Print and shaded views of the part. All mm, measured from the part's lowest x, y and z. A direction names the side the tool comes from. Coordinates: 2 decimals unless noted, no trailing zeros. Loops run counter-clockwise (first coordinate to the right, second up) from the corner with the lowest first, then second, coordinate; pieces in that order, holes last. Notation, with made-up numbers: M -2.5,-37 L 29.5,-37 A24 cw 29.5,-4 Z; hole C 15,4.25 d5. An arc over 180 degrees is marked long. Use a Markdown table: item, result. Add a question column.
1) Wall check: probe 1 along Y at (x, z) = (51, 8.5); probe 2 along Y at (x, z) = (49.25, 8.5); probe 3 along Z at (x, y) = (3.5, 7.25). Give the ranges that are in metal, low to high. Write a range as from..to.
2) Pull direction Z, two halves, no side cores. Call the marked faces 4, 5 and 6: released by +Z, released by -Z, zero draft, split by the parting line, or undercut.
3) Band-saw the part on B-B (y = 47.69). List the corners of the cut face in (x, z).
4) Band-saw the part on D-D (z = 16.25). List the corners of the cut face in (x, y), plus the area to 3 significant figures.
5) Pin check, flat tips, straight feed: pin 1 Ø5 at (y, z) = (42, 3) entering from -X; pin 2 Ø9 at (x, z) = (13, 10) entering from +Y; pin 3 Ø2 at (x, y) = (7, 7.5) entering from +Z; pin 4 Ø4 at (y, z) = (31, 8.5) entering from -X. Stop position of each tip, or through.
6) Tool access for the marked faces 1, 2 and 3: list every direction of +Z, -Z, +X, -X, +Y, -Y with a clear straight run to the whole face (end or side of a thin tool).
7) Band-saw the part on A-A (z = 8.5). List the corners of the cut face in (x, y), plus the area to 3 significant figures.
8) Band-saw the part on C-C (x = 3.5). List the corners of the cut face in (y, z).
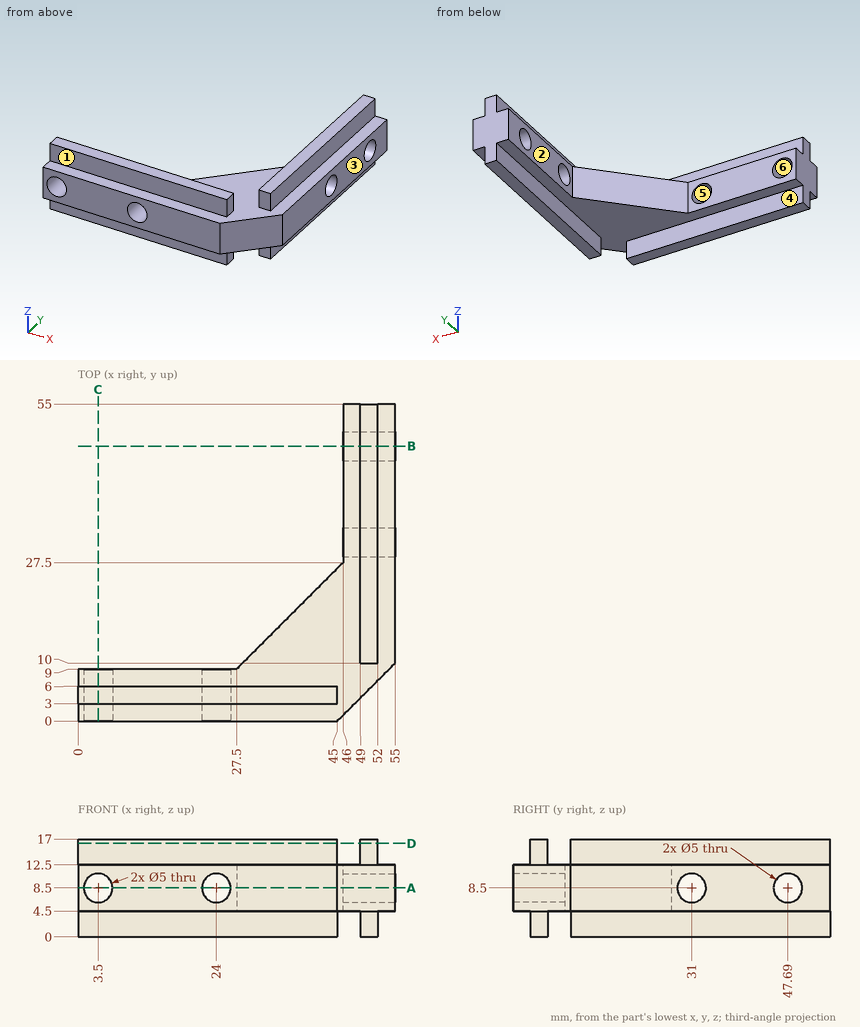
Entries:
| question | item | result |
|---|---|---|
| 1 | probe 1 | 6..28.5, 33.5..45.19, 50.19..55 |
| 1 | probe 2 | 4.25..28.5, 33.5..45.19, 50.19..55 |
| 1 | probe 3 | 4.5..6, 11..12.5 |
| 2 | face 4 | zero draft |
| 2 | face 5 | undercut |
| 2 | face 6 | undercut |
| 3 | outline | M 46,4.5 L 49,4.5 L 49,0 L 52,0 L 52,4.5 L 55,4.5 L 55,6 L 46,6 Z; M 46,11 L 55,11 L 55,12.5 L 52,12.5 L 52,17 L 49,17 L 49,12.5 L 46,12.5 Z |
| 4 | outline | M 0,3 L 45,3 L 45,6 L 0,6 Z; M 49,10 L 52,10 L 52,55 L 49,55 Z |
| 4 | area | 270 mm2 |
| 5 | pin 1 | x = 46 |
| 5 | pin 2 | y = 9 |
| 5 | pin 3 | z = 12.5 |
| 5 | pin 4 | through |
| 6 | face 1 | +Z, +X, -X, -Y |
| 6 | face 2 | +Z, -Z, -X, +Y |
| 6 | face 3 | +Z, -Z, +X, +Y, -Y |
| 7 | outline | M 0,0 L 1,0 L 1,9 L 0,9 Z; M 6,0 L 21.5,0 L 21.5,9 L 6,9 Z; M 26.5,0 L 45,0 L 55,10 L 55,28.5 L 46,28.5 L 46,27.5 L 27.5,9 L 26.5,9 Z; M 46,33.5 L 55,33.5 L 55,45.19 L 46,45.19 Z; M 46,50.19 L 55,50.19 L 55,55 L 46,55 Z |
| 7 | area | 850 mm2 |
| 8 | outline | M 0,4.5 L 3,4.5 L 3,0 L 6,0 L 6,4.5 L 9,4.5 L 9,6 L 0,6 Z; M 0,11 L 9,11 L 9,12.5 L 6,12.5 L 6,17 L 3,17 L 3,12.5 L 0,12.5 Z |
